from build123d import *

# Parameters (mm, degrees)
SKETCH_1_W      = 25
SKETCH_1_H      = 24
SKETCH_1_R      = 1
EXTRUDE_1_DEPTH = 1
SKETCH_3_R      = 6.5
EXTRUDE_4_DEPTH = 16
EXTRUDE_5_DEPTH = 3.5
SKETCH_5_R      = 5
EXTRUDE_6_DEPTH = 2
FILLET_1_R      = 5
SKETCH_10_R     = 1.5
EXTRUDE_7_DEPTH = 1
FILLET_2_R      = 1


# Some blends are built 0.0001 mm under size
with BuildPart() as part:
    # Эскиз1 → Бобышка-Вытянуть1 (new body)
    with BuildSketch(Plane(origin=(0, 0, 0), x_dir=(1, 0, 0), z_dir=(0, 1, 0))):
        with Locations((-12.5, 12)):
            Rectangle(SKETCH_1_W, SKETCH_1_H)
        with Locations(Location((-23, 22, 0), (0, 0, 270))):
            Circle(SKETCH_1_R, mode=Mode.SUBTRACT)
        with Locations(Location((-2, 22, 0), (0, 0, 270))):
            Circle(SKETCH_1_R, mode=Mode.SUBTRACT)
        with Locations(Location((-23, 8.5, 0), (0, 0, 270))):
            Circle(SKETCH_1_R, mode=Mode.SUBTRACT)
        with Locations(Location((-2, 8.5, 0), (0, 0, 270))):
            Circle(SKETCH_1_R, mode=Mode.SUBTRACT)
    extrude(amount=EXTRUDE_1_DEPTH)

    # Эскиз3 → Бобышка-Вытянуть4 (add)
    with BuildSketch(Plane(origin=(0, 1, 0), x_dir=(1, 0, 0), z_dir=(0, 1, 0))):
        with Locations(Location((-12.5, 15.5, 0), (0, 0, 270))):
            Circle(SKETCH_3_R)
    extrude(amount=EXTRUDE_4_DEPTH)

    # Эскиз3<5> → Бобышка-Вытянуть5 (add)
    with BuildSketch(Plane(origin=(0, 1, 0), x_dir=(1, 0, 0), z_dir=(0, 1, 0))):
        with BuildLine():
            Line((-19, 21.5), (-19, 9.5))
            ThreePointArc((-19, 9.5), (-18.853553391, 9.146446609), (-18.5, 9))
            Line((-18.5, 9), (-6.5, 9))
            ThreePointArc((-6.5, 9), (-6.146446609, 9.146446609), (-6, 9.5))
            Line((-6, 9.5), (-6, 21.5))
            ThreePointArc((-6, 21.5), (-6.146446609, 21.853553391), (-6.5, 22))
            Line((-6.5, 22), (-18.5, 22))
            ThreePointArc((-18.5, 22), (-18.853553391, 21.853553391), (-19, 21.5))
        make_face()
    extrude(amount=EXTRUDE_5_DEPTH)

    # Эскиз5 → Бобышка-Вытянуть6 (add)
    with BuildSketch(Plane(origin=(0, 17, 0), x_dir=(1, 0, 0), z_dir=(0, 1, 0))):
        with Locations(Location((-12.5, 15.5, 0), (0, 0, 270))):
            Circle(SKETCH_5_R)
    extrude(amount=EXTRUDE_6_DEPTH)

    # Скругление1
    # the kernel refuses this fillet: 5 mm, written as the material it takes off along each edge
    with BuildSketch(Plane(origin=(-12.5, 19, -15.5), x_dir=(0, 0, 1), z_dir=(-1, 0, 0))) as fillet_1_piece_1:
        with BuildLine():
            CenterArc((1, -5), FILLET_1_R, 36.869897646, 53.130102354)
            Line((1, 0), (1, 0.1))
            Line((1, 0.1), (5, 0.1))
            Line((5, 0.1), (5.1, 0))
            ThreePointArc((5.1, 0), (5.1, -1), (5.08, -1.94))
            Line((5.08, -1.94), (5, -2))
        make_face()
    revolve(axis=Axis((-12.5, 19, -15.5), (0, 1, 0)), mode=Mode.SUBTRACT)

    # Эскиз10 → Бобышка-Вытянуть7 (add)
    with BuildSketch(Plane.XZ):
        with Locations(Location((-21.5, -15.5, 0), (0, 0, 90))):
            Circle(SKETCH_10_R)
        with Locations(Location((-3.5, -15.5, 0), (0, 0, 90))):
            Circle(SKETCH_10_R)
    extrude(amount=EXTRUDE_7_DEPTH)

    # Скругление2
    fillet_2_edges = [part.edges().sort_by_distance(p)[0] for p in [
        (-21.5, -1, -17),
        (-3.5, -1, -17),
    ]]
    fillet(fillet_2_edges, radius=FILLET_2_R - 0.0001)  # a hair under: the kernel refuses the full size


solid = part.part
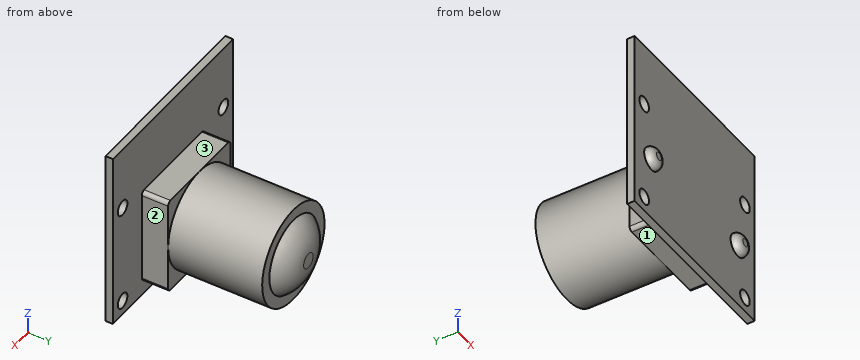
Could you check a few things on this model? Use its own coordinates, in mm. Face numbers are marked on the shaded views. A direction names the side the tool comes from. Give positions to 0.01 mm unless a question says otherwise; leave off trailing zeros. Order: outer loops, then holes, each group sorted by start corner. A loop starts at its lowest first (then second) coordinate and runs counter-clockwise, first axis right, second up.
1. Suppose I cut it at C-C (x = -22.5). State how many separate pieces and enclosed holes the cut face has, plus the area to 3 significant figures.
Answers below:
separate pieces: 3
enclosed holes: 0
area: 22.1 mm2
2. Suppose I cut it at A-A (z = -8.5). Write out the boundary of the cut face in (x, y).
Answers below:
outline: (-25, 0) - (-24, 0) - (-24, 1) - (-25, 1) - close; (-22, 0) - (-3, 0) - (-3, 1) - (-22, 1) - close; (-1, 0) - (0, 0) - (0, 1) - (-1, 1) - close
3. Which directions (+Z, -Z, +X, -X, +Y, -Y) give clear straight access to the entire face, cutting with the end or side of a thin tool? Please do the marked faces 1, 2 and 3.
Answers below:
face 1: -Z, +X, -X, +Y
face 2: +Z, -Z, +X, +Y
face 3: +Z, +X, -X, +Y
4. For pin 1 (3 mm diameter, centred on x = -21.5, z = -5.5, fed in from -Y); pin 2 (1 mm diameter, centred on y = 2.5, z = -19.5, fed in from +X); pin 3 (5 mm diameter, centred on x = -4.5, y = 13.5, fed in from -Z); pin 4 (1.6 mm diameter, centred on x = -2, z = -8.5, fed in from +Y), each with a flat end and sliding along its axis, tell me the tip position at first contact or that it passes through.
Answers below:
pin 1: stops at y = 0
pin 2: stops at x = -6
pin 3: stops at z = -18.96
pin 4: passes through
5. Suppose I cut it at B-B (y = 5). Write out the boundary of the cut face in (x, z).
Answers below:
outline: circle Ø13 at (-12.5, -15.5)
6. I need wall thicknesses on L1, parallel to X at y = 0.5, z = -8.5; L2, parallel to Y at x = -18, z = -2; L3, parallel to X at y = 12.75, z = -15.25. Which ranges of each line are inside material? Lowest first, please.
Answers below:
L1: x = -25 to -24, -22 to -3, -1 to 0
L2: y = 0 to 1
L3: x = -19 to -6
